Design review of the part built by this model. Coordinates are the model's own, in mm. A direction names the side the tool comes from. Give positions to 0.01 mm unless a question says otherwise; leave off trailing zeros. Loops run counter-clockwise (first coordinate to the right, second up) from the corner with the lowest first, then second, coordinate; pieces in that order, holes last. Notation, with made-up numbers: (57, -12.5) -> (111, -12.5) arc R24 cw to (111, 17.5) -> close; hole circle Ø3 at (-12.75, -20). An arc over 180 degrees is marked (long way). Use CSV: the item, a comma, the result in double quotes. Start each with the question number.
Item 1: Clearance check with flat-ended pins moving along their axes: pin 1 (6 mm diameter, centred on y = -6.5, z = -2, fed in from +X); pin 2 (2 mm diameter, centred on x = -29.5, z = 17.5, fed in from +Y); pin 3 (4 mm diameter, centred on y = 9, z = -0.74, fed in from +X). State where each tip first meets the part, or that it passes through.
Item 2: We need section D-D (y = -28). State the section outline as (x, z) points.
Item 3: Wall thickness on line 1 along Y through (x, z) = (-8, -1); line 2 along Y through (x, z) = (-56.5, 11); line 3 along Y through (x, z) = (-10, 5): over which ranges is each line inside the solid? List them lowest first. Write a range as from..to.
Item 4: For faces 4 (the face through (-31, 61.588, -13)), 5 (the face through (-37, -32, 0)), 6 (the face through (-8, 14, -10.737)), 7 (the face through (-5.817, -17, -1)), 8 (the face through (-6.27, 23.48, -0.41)), list the 3-axis set-ups (+Z, -Z, +X, -X, +Y, -Y) from which the entire face can be reached by the end or side of a thin tool; tool diameter is ignored.
Item 5: We need section C-C (x = -46). State the section outline as (y, z) points, plus the area to 3 significant figures.
Item 6: We need section B-B (z = -12). State the section outline as (x, y) points.
Item 7: The part is to be moulded in two halves that separate along X. For faces 1 (the face through (-43, 58, 7)), 2 (the face through (-15.5, 65, -1.1)), 3 (the face through (-2.817, 15, -1)), say which applies: +X half, -X half, draft (parallel to the pull), parting line (faces both ways), or undercut.
Item 8: We need section A-A (y = 21). State the section outline as (x, z) points, plus the area to 4 significant figures.
Autodesk Inventor part; units mm, degrees
ref_plane "YZ Plane" through (0, 0, 0) normal (1, 0, 0) x (0, 1, 0)
ref_plane "XZ Plane" through (0, 0, 0) normal (0, 1, 0) x (-1, 0, 0)
ref_plane "XY Plane" through (0, 0, 0) normal (0, 0, 1) x (1, 0, 0)
sketch "Sketch1" plane through (0, 0, 0) normal (0, 1, 0) x (-1, 0, 0)
  line L0 (5.8173, 9.2628) -> (2.8173, 9.2628)
  line L1 (2.8173, 9.2628) -> (2.8173, -10.7372)
  line L2 (2.8173, -10.7372) -> (5.8173, -10.7372)
  line L3 (5.8173, -10.7372) -> (5.8173, 9.2628)
  point P0 (0, 0)
  dimension "d0" = 20
  dimension "d1" = 3
extrude "Extrusion1" add sketch "Sketch1" along normal blind 30
sketch "Sketch2" plane through (-2.8173, 0, 9.2628) normal (1, 0, 0) x (0, 0, -1)
  circle A0 centre (10, 21) radius 2.5
  circle A1 centre (10, 9) radius 2.5
  line L0 (0, 30) -> (20, 30)
  line L1 (0, 0) -> (20, 0)
  line L2 (10, 30) -> (10, 21) construction
  line L3 (10, 9) -> (10, 0) construction
  point P0 (9.2628, 0)
  dimension "d4" = 5
  dimension "d5" = 5
  dimension "d41" = 12
sketch "Sketch3" plane through (-5.8173, 0, -10.7372) normal (-1, 0, 0) x (0, 0, 1)
  line L0 (0, 65) -> (20, 65)
  line L1 (20, 65) -> (20, -35)
  line L2 (20, -35) -> (0, -35)
  line L3 (0, -35) -> (0, 65)
  line L4 (20, 0) -> (20, 30)
  line L5 (0, 0) -> (0, 30)
  line L6 (0, 30) -> (20, 30)
  line L7 (0, 0) -> (20, 0)
  point P0 (10.7372, 0)
  dimension "d9" = 35
  dimension "d10" = 35
extrude "Extrusion2" add sketch "Sketch3" along normal blind 6
sketch "Sketch4" plane through (-5.8173, 65, 9.2628) normal (0, 1, 0) x (1, 0, 0)
  line L0 (-56, 35) -> (-6, 35)
  line L1 (-6, 35) -> (-6, -15)
  line L2 (-6, -15) -> (-56, -15)
  line L3 (-56, -15) -> (-56, 35)
  line L4 (-6, 0) -> (-6, 20)
  line L5 (0, 20) -> (-6, 20)
  line L6 (-6, 10) -> (-56, 10) construction
  line L7 (-31, 35) -> (-31, 10) construction
  line L8 (-31, -15) -> (-31, 10) construction
  line L9 (-10, 31) -> (-52, 31)
  line L10 (-52, 31) -> (-52, -11)
  line L11 (-52, -11) -> (-10, -11)
  line L12 (-10, -11) -> (-10, 31)
  point P0 (5.8173, 9.2628)
  dimension "d13" = 50
  dimension "d14" = 50
  dimension "d16" = 4
extrude "Extrusion3" add sketch "Sketch4" against normal blind 7
sketch "Sketch5" plane through (-5.8173, 58, 9.2628) normal (0, -1, 0) x (1, 0, 0)
  line L0 (-56, 15) -> (-56, -35)
  line L1 (-56, -35) -> (-6, -35)
  line L2 (-6, -35) -> (-6, -20)
  line L3 (-6, 0) -> (-6, -20)
  line L4 (-6, 0) -> (-6, 15)
  line L5 (-6, 15) -> (-56, 15)
  line L6 (-10, 11) -> (-10, -31)
  line L7 (-10, -31) -> (-52, -31)
  line L8 (-52, -31) -> (-52, 11)
  line L9 (-52, 11) -> (-10, 11)
  point P0 (5.8173, -9.2628)
extrude "Extrusion4" add sketch "Sketch5" along normal blind 90 contours L5 L4 L3 L2 L1 L0 | L6 L7 L8 L9
sketch "Sketch6" plane through (-5.8173, -32, 9.2628) normal (0, -1, 0) x (1, 0, 0)
  line L0 (-10, 11) -> (-10, -31)
  line L1 (-52, 11) -> (-10, 11)
  line L2 (-52, -31) -> (-52, 11)
  line L3 (-10, -31) -> (-52, -31)
  line L4 (-6, 15) -> (-56, 15)
  line L5 (-56, 15) -> (-56, -35)
  line L6 (-56, -35) -> (-6, -35)
  line L7 (-6, -35) -> (-6, -20)
  line L8 (-6, 0) -> (-6, -20)
  line L9 (-6, 0) -> (-6, 15)
  point P0 (5.8173, -9.2628)
extrude "Extrusion5" add sketch "Sketch6" along normal blind 7
extrude "Extrusion6" cut sketch "Sketch2" against normal blind 7
sketch "Sketch7" plane through (-5.8173, -32, 9.2628) normal (0, -1, 0) x (1, 0, 0)
  circle A0 centre (-31.392, -9.2628) radius 20
  line L0 (-10, 11) -> (-52, 11)
  line L1 (-52, 11) -> (-52, -31)
  line L2 (-52, -31) -> (-10, -31)
  line L3 (-10, -31) -> (-10, 11)
  line L4 (-6, 15) -> (-56, 15)
  line L5 (-56, 15) -> (-56, -35)
  line L6 (-56, -35) -> (-6, -35)
  line L7 (-6, -35) -> (-6, 15)
  line L8 (-10, 11) -> (-10, -31)
  line L9 (-10, -31) -> (-52, -31)
  line L10 (-52, -31) -> (-52, 11)
  line L11 (-52, 11) -> (-10, 11)
  point P0 (5.8173, -9.2628)
  dimension "d25" = 40
extrude "Extrusion7" add sketch "Sketch7" along normal blind 7 contours L3 L2 L1 L0
sketch "Sketch8" plane through (-5.8173, 58, 9.2628) normal (0, 1, 0) x (1, 0, 0)
  circle A0 centre (-21, 20) radius 5
  line L0 (-46, -5) -> (-31, -5)
  line L1 (-31, -5) -> (-31, 10)
  line L2 (-31, 10) -> (-46, 10)
  line L3 (-46, 10) -> (-46, -5)
  line L4 (-6, 35) -> (-56, 35)
  line L5 (-6, 20) -> (-6, 35)
  line L6 (-56, -15) -> (-6, -15)
  line L7 (-56, 35) -> (-56, -15)
  circle A1 centre (-21, 20) radius 4.5053
  line L8 (-42.9073, -3.8349) -> (-32.3073, -3.8349)
  line L9 (-32.3073, -3.8349) -> (-32.3073, 9.1651)
  line L10 (-32.3073, 9.1651) -> (-42.9073, 9.1651)
  line L11 (-42.9073, 9.1651) -> (-42.9073, -3.8349)
  point P0 (5.8173, 9.2628)
  dimension "d28" = 15
  dimension "d29" = 15
  dimension "d30" = 10
  dimension "d31" = 15
  dimension "d32" = 15
  dimension "d33" = 10
  dimension "d34" = 10
  dimension "d35" = 10.6
  dimension "d36" = 13
extrude "Extrusion8" add sketch "Sketch8" along normal blind 1
sketch "Sketch10" plane through (-26.8173, 59, -10.7372) normal (0, 1, 0) x (1, 0, 0)
  circle A0 centre (0, 0) radius 4.5053
  circle A1 centre (0, 0) radius 5
  point P0 (26.8173, -10.7372)
extrude "Extrusion9" add sketch "Sketch10" along normal blind 2.5875
properties part number "camera" material "PAEK Plastic"
Results found:
1,pin 1,"x = -5.82"
1,pin 2,"y = 58"
1,pin 3,"x = -9.82"
2,outline,"(-61.82, -25.74) -> (-11.82, -25.74) -> (-11.82, -10.74) -> (-5.82, -10.74) -> (-5.82, 9.26) -> (-11.82, 9.26) -> (-11.82, 24.26) -> (-61.82, 24.26) -> close"
3,line 1,"-35..6.51, 11.49..18.51, 23.49..65"
3,line 2,"-39..58"
3,line 3,"-35..65"
4,face 4,"+Y"
4,face 5,"-Y"
4,face 6,"-Z, +X, +Y, -Y"
4,face 7,"+Z, -Z, +X, -Y"
4,face 8,"+X"
5,outline,"(-39, -25.74) -> (65, -25.74) -> (65, -21.74) -> (58, -21.74) -> (58, -0.74) -> (59, -0.74) -> (59, 0.1) -> (58, 0.1) -> (58, 13.1) -> (59, 13.1) -> (59, 14.26) -> (58, 14.26) -> (58, 20.26) -> (65, 20.26) -> (65, 24.26) -> (-39, 24.26) -> (-39, 17.96) -> (-32, 17.96) -> (-32, -17.96) -> (-39, -17.96) -> close"
5,area,"4,660 mm²"
6,outline,"(-61.82, -39) -> (-53.21, -39) -> (-53.21, -32) -> (-21.21, -32) -> (-21.21, -39) -> (-11.82, -39) -> (-11.82, 65) -> (-15.82, 65) -> (-15.82, 58) -> (-21.98, 58) -> (-21.98, 61.59) -> (-22.49, 61.59) -> (-22.49, 58) -> (-31.14, 58) -> (-31.14, 61.59) -> (-31.66, 61.59) -> (-31.66, 58) -> (-57.82, 58) -> (-57.82, 65) -> (-61.82, 65) -> close"
7,face 1,"undercut"
7,face 2,"draft"
7,face 3,"+X half"
8,outline,"(-61.82, -25.74) -> (-11.82, -25.74) -> (-11.82, -10.74) -> (-2.82, -10.74) -> (-2.82, -3.24) -> (-9.82, -3.24) -> (-9.82, 1.76) -> (-2.82, 1.76) -> (-2.82, 9.26) -> (-11.82, 9.26) -> (-11.82, 24.26) -> (-61.82, 24.26) -> close"
8,area,"2,645 mm²"
